Geometry: final body of the model. Coordinates: model frame, mm. Face numbers are marked on the shaded views. Give positions to 0.01 mm unless a question says otherwise; leave off trailing zeros. Write each loop counter-clockwise with the first axis right and the second up, starting at its lowest first coordinate (ties: lowest second). Pieces come first, ordered by that corner, then holes. Notation, with made-up numbers: (-34.75, -31) - (-2.75, -31) arc R22 ccw to (-2.75, -8) - close; hole circle Ø3 at (-26, 34). An arc over 180 degrees is marked (long way). Use CSV: the item, a comma, the result in double quotes. Start each with the question number.
(1) Section C-C on z = -36. Output: boundary loops of the cut face in (x, y), and give its area (3 significant figures).
(2) Draft query along Z for the marked faces 1 and 2. Return one class per face: released by +Z, released by -Z, zero draft, split by the parting line, or undercut.
(3) Section A-A on z = -1. Output: boundary loops of the cut face in (x, y), and give its area (3 significant figures).
(4) First-contact query: pin 1 Ø16 at (x, z) = (-97.5, -47) entering from +Y; pin 2 Ø3.5 at (x, z) = (-100, -71) entering from -Y; pin 3 Ø6.5 at (x, z) = (-92, -43.5) entering from +Y; pin 4 Ø5 at (x, z) = (-98.5, -71.5) entering from -Y. Flat tips, straight axial feed; report the tip coordinate or a pass-through.
(5) Line query: probe 1 along X at (y, z) = (-0.15, -71); probe 2 along X at (y, z) = (0.15, -45); probe 3 along Z at (x, y) = (-100, 0.1). Output: solid intervals per line, ascending. Write a range as [from, to].
(6) Section B-B on x = -1. Output: boundary loops of the cut face in (y, z), and give its area (3 significant figures).
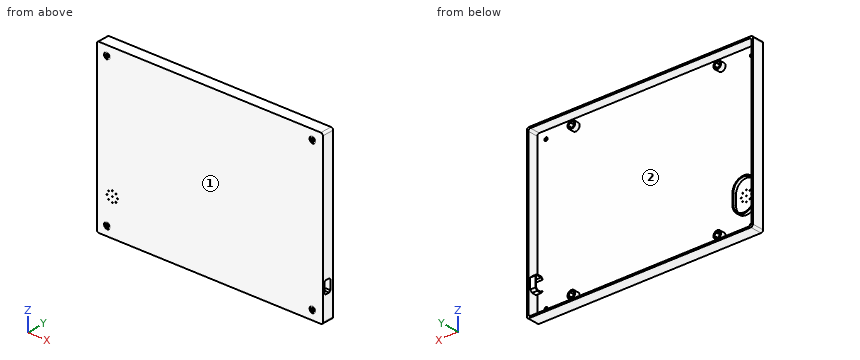
from build123d import *

# Parameters (mm, degrees)
EXTRUDE_1_DEPTH                 = 1
EXTRUDE_1_DEPTH_BACK            = 0.5
SKETCH_1_W                      = 220
SKETCH_1_H                      = 160
SKETCH_2_R                      = 3.75
EXTRUDE_2_DEPTH                 = 5
CUT_EXTRUDE_5_REACH             = 138.17
SKETCH_3_R                      = 1.6
CUT_EXTRUDE_5_DIRECTION_2_DEPTH = 137.169930601
CUT_EXTRUDE_START               = -0.5
SKETCH_4_R                      = 3
CUT_EXTRUDE_7_DEPTH             = 0.5
SKETCH_5_W                      = 220
SKETCH_5_H                      = 160
SKETCH_5_W_2                    = 217
SKETCH_5_H_2                    = 157
EXTRUDE_3_DEPTH                 = 10
FILLET_1_R                      = 2
FILLET_2_R                      = 2
FILLET_3_R                      = 2
CUT_EXTRUDE_8_REACH             = 236.352
CUT_EXTRUDE_8_DIRECTION_2_DEPTH = 235.352298901
EXTRUDE_4_DEPTH                 = 5
EXTRUDE_5_DEPTH                 = 3
CUT_EXTRUDE_9_REACH             = 138.382
SKETCH_10_R                     = 0.5


with BuildPart() as part:
    # 草图1 → 凸台-拉伸1 (new, two sides: drawn at the far end of the back side and taken through both)
    with BuildSketch(Plane(origin=(0, 0, 0), x_dir=(1, 0, 0), z_dir=(0, 1, 0)).offset(-EXTRUDE_1_DEPTH_BACK)):
        Rectangle(SKETCH_1_W, SKETCH_1_H)
    extrude(amount=EXTRUDE_1_DEPTH + EXTRUDE_1_DEPTH_BACK)

    # 草图2 → 凸台-拉伸2 (add)
    # profile 1 of 4: a face of its own
    with BuildSketch(Plane(origin=(0, 1, 0), x_dir=(1, 0, 0), z_dir=(0, 1, 0))):
        with Locations(Location((-71, 71, 0), (0, 0, 270))):
            Circle(SKETCH_2_R)
        Polygon((-69.614359354, 68.6), (-68.228718708, 71), (-69.614359354, 73.4), (-72.385640646, 73.4), (-73.771281292, 71), (-72.385640646, 68.6), align=None, mode=Mode.SUBTRACT)
    # profile 2 of 4: a face of its own
    with BuildSketch(Plane(origin=(0, 1, 0), x_dir=(1, 0, 0), z_dir=(0, 1, 0))):
        with Locations(Location((71, 71, 0), (0, 0, 90))):
            Circle(SKETCH_2_R)
        Polygon((72.385640646, 68.6), (69.614359354, 68.6), (68.228718708, 71), (69.614359354, 73.4), (72.385640646, 73.4), (73.771281292, 71), align=None, mode=Mode.SUBTRACT)
    # profile 3 of 4: a face of its own
    with BuildSketch(Plane(origin=(0, 1, 0), x_dir=(1, 0, 0), z_dir=(0, 1, 0))):
        with Locations(Location((71, -71, 0), (0, 0, 270))):
            Circle(SKETCH_2_R)
        Polygon((69.614359354, -68.6), (68.228718708, -71), (69.614359354, -73.4), (72.385640646, -73.4), (73.771281292, -71), (72.385640646, -68.6), align=None, mode=Mode.SUBTRACT)
    # profile 4 of 4: a face of its own
    with BuildSketch(Plane(origin=(0, 1, 0), x_dir=(1, 0, 0), z_dir=(0, 1, 0))):
        with Locations(Location((-71, -71, 0), (0, 0, 90))):
            Circle(SKETCH_2_R)
        Polygon((-72.385640646, -68.6), (-69.614359354, -68.6), (-68.228718708, -71), (-69.614359354, -73.4), (-72.385640646, -73.4), (-73.771281292, -71), align=None, mode=Mode.SUBTRACT)
    extrude(amount=EXTRUDE_2_DEPTH)

    # 草图3 → 切除-拉伸5 (cut, up to next)
    with BuildSketch(Plane.XZ.offset(0.5), mode=Mode.PRIVATE) as cut_extrude_5_sk1:
        with Locations(Location((-100, -71, 0), (0, 0, 90))):
            Circle(SKETCH_3_R)
    cut_extrude_5_tool1 = extrude(cut_extrude_5_sk1.sketch, amount=-CUT_EXTRUDE_5_REACH, mode=Mode.PRIVATE) & part.part
    # 草图3 → 切除-拉伸5 (cut, up to next)
    with BuildSketch(Plane.XZ.offset(0.5), mode=Mode.PRIVATE) as cut_extrude_5_sk2:
        with Locations(Location((100, -71, 0), (0, 0, 90))):
            Circle(SKETCH_3_R)
    cut_extrude_5_tool2 = extrude(cut_extrude_5_sk2.sketch, amount=-CUT_EXTRUDE_5_REACH, mode=Mode.PRIVATE) & part.part
    # 草图3 → 切除-拉伸5 (cut, up to next)
    with BuildSketch(Plane.XZ.offset(0.5), mode=Mode.PRIVATE) as cut_extrude_5_sk3:
        with Locations(Location((100, 71, 0), (0, 0, 90))):
            Circle(SKETCH_3_R)
    cut_extrude_5_tool3 = extrude(cut_extrude_5_sk3.sketch, amount=-CUT_EXTRUDE_5_REACH, mode=Mode.PRIVATE) & part.part
    # 草图3 → 切除-拉伸5 (cut, up to next)
    with BuildSketch(Plane.XZ.offset(0.5), mode=Mode.PRIVATE) as cut_extrude_5_sk4:
        with Locations(Location((-100, 71, 0), (0, 0, 90))):
            Circle(SKETCH_3_R)
    cut_extrude_5_tool4 = extrude(cut_extrude_5_sk4.sketch, amount=-CUT_EXTRUDE_5_REACH, mode=Mode.PRIVATE) & part.part
    add(cut_extrude_5_tool1.solids().sort_by_distance((-100, -0.5, -71))[0], mode=Mode.SUBTRACT)
    add(cut_extrude_5_tool2.solids().sort_by_distance((100, -0.5, -71))[0], mode=Mode.SUBTRACT)
    add(cut_extrude_5_tool3.solids().sort_by_distance((100, -0.5, 71))[0], mode=Mode.SUBTRACT)
    add(cut_extrude_5_tool4.solids().sort_by_distance((-100, -0.5, 71))[0], mode=Mode.SUBTRACT)

    # 草图3 → 切除-拉伸5 direction 2 (cut)
    with BuildSketch(Plane.XZ.offset(0.5)):
        with Locations(Location((-100, -71, 0), (0, 0, 90))):
            Circle(SKETCH_3_R)
        with Locations(Location((100, -71, 0), (0, 0, 90))):
            Circle(SKETCH_3_R)
        with Locations(Location((100, 71, 0), (0, 0, 90))):
            Circle(SKETCH_3_R)
        with Locations(Location((-100, 71, 0), (0, 0, 90))):
            Circle(SKETCH_3_R)
    extrude(amount=CUT_EXTRUDE_5_DIRECTION_2_DEPTH, mode=Mode.SUBTRACT)

    # 草图4 → 切除-拉伸7 (cut)
    with BuildSketch(Plane(origin=(0, 0, 0), x_dir=(1, 0, 0), z_dir=(0, 1, 0)).offset(CUT_EXTRUDE_START)):
        with Locations(Location((-100, 71, 0), (0, 0, 270))):
            Circle(SKETCH_4_R)
        with Locations(Location((100, 71, 0), (0, 0, 90))):
            Circle(SKETCH_4_R)
        with Locations(Location((100, -71, 0), (0, 0, 270))):
            Circle(SKETCH_4_R)
        with Locations(Location((-100, -71, 0), (0, 0, 90))):
            Circle(SKETCH_4_R)
    extrude(amount=CUT_EXTRUDE_7_DEPTH, mode=Mode.SUBTRACT)

    # 草图5 → 凸台-拉伸3 (add)
    with BuildSketch(Plane(origin=(0, 1, 0), x_dir=(1, 0, 0), z_dir=(0, 1, 0))):
        Rectangle(SKETCH_5_W, SKETCH_5_H)
        Rectangle(SKETCH_5_W_2, SKETCH_5_H_2, mode=Mode.SUBTRACT)
    extrude(amount=EXTRUDE_3_DEPTH)

    # 圆角1
    fillet_1_edges = [part.edges().sort_by_distance(p)[0] for p in [
        (-110, 5.25, -80),
    ]]
    fillet(fillet_1_edges, radius=FILLET_1_R)

    # 圆角2
    fillet_2_edges = [part.edges().sort_by_distance(p)[0] for p in [
        (-108.5, 6, -78.5),
    ]]
    fillet(fillet_2_edges, radius=FILLET_2_R)

    # 圆角3
    fillet_3_edges = [part.edges().sort_by_distance(p)[0] for p in [
        (108.5, 6, 78.5),
        (108.5, 6, -78.5),
        (-108.5, 6, 78.5),
        (110, 5.25, 80),
        (-110, 5.25, 80),
        (110, 5.25, -80),
    ]]
    fillet(fillet_3_edges, radius=FILLET_3_R)

    # 草图7 → 切除-拉伸8 (cut, up to next)
    with BuildSketch(Plane(origin=(110, 0, 0), x_dir=(0, 0, -1), z_dir=(1, 0, 0)), mode=Mode.PRIVATE) as cut_extrude_8_sk1:
        Polygon((45.435952693, 8), (54.607525568, 8), (56.02173913, 6.585786438), (56.02173913, 2.414213562), (54.607525568, 1), (45.435952693, 1), (44.02173913, 2.414213562), (44.02173913, 6.585786438), align=None)
    cut_extrude_8_tool1 = extrude(cut_extrude_8_sk1.sketch, amount=-CUT_EXTRUDE_8_REACH, mode=Mode.PRIVATE) & part.part
    add(cut_extrude_8_tool1.solids().sort_by_distance((110, 4.5, -50.021739))[0], mode=Mode.SUBTRACT)

    # 草图7 → 切除-拉伸8 direction 2 (cut)
    with BuildSketch(Plane(origin=(110, 0, 0), x_dir=(0, 0, -1), z_dir=(1, 0, 0))):
        Polygon((45.435952693, 8), (54.607525568, 8), (56.02173913, 6.585786438), (56.02173913, 2.414213562), (54.607525568, 1), (45.435952693, 1), (44.02173913, 2.414213562), (44.02173913, 6.585786438), align=None)
    extrude(amount=CUT_EXTRUDE_8_DIRECTION_2_DEPTH, mode=Mode.SUBTRACT)

    # 草图8 → 凸台-拉伸4 (add)
    with BuildSketch(Plane.ZY.offset(-108.5)):
        Polygon((-44.435952693, 1), (-43.02173913, 2.414213562), (-43.02173913, 7), (-45.02173913, 9), (-55.02173913, 9), (-57.02173913, 7), (-57.02173913, 2.414213562), (-55.607525568, 1), (-54.607525568, 1), (-56.02173913, 2.414213562), (-56.02173913, 6.585786438), (-54.607525568, 8), (-45.435952693, 8), (-44.02173913, 6.585786438), (-44.02173913, 2.414213562), (-45.435952693, 1), align=None)
    extrude(amount=EXTRUDE_4_DEPTH)

    # 草图9 → 凸台-拉伸5 (add)
    with BuildSketch(Plane(origin=(0, 1, 0), x_dir=(1, 0, 0), z_dir=(0, 1, 0))):
        with BuildLine():
            Line((-84, 50), (-84, 40))
            ThreePointArc((-84, 40), (-95, 29), (-106, 40))
            Line((-106, 40), (-106, 50))
            ThreePointArc((-106, 50), (-95, 61), (-84, 50))
        make_face()
        with BuildLine():
            Line((-85, 50), (-85, 40))
            ThreePointArc((-85, 40), (-95, 30), (-105, 40))
            Line((-105, 40), (-105, 50))
            ThreePointArc((-105, 50), (-95, 60), (-85, 50))
        make_face(mode=Mode.SUBTRACT)
    extrude(amount=EXTRUDE_5_DEPTH)

    # 草图10 → 切除-拉伸9 (cut, up to next)
    with BuildSketch(Plane(origin=(0, 1, 0), x_dir=(1, 0, 0), z_dir=(0, 1, 0)), mode=Mode.PRIVATE) as cut_extrude_9_sk1:
        with Locations(Location((-95, 45, 0), (0, 0, 270))):
            Circle(SKETCH_10_R)
    cut_extrude_9_tool1 = extrude(cut_extrude_9_sk1.sketch, amount=-CUT_EXTRUDE_9_REACH, mode=Mode.PRIVATE) & part.part
    # 草图10 → 切除-拉伸9 (cut, up to next)
    with BuildSketch(Plane(origin=(0, 1, 0), x_dir=(1, 0, 0), z_dir=(0, 1, 0)), mode=Mode.PRIVATE) as cut_extrude_9_sk2:
        with Locations(Location((-100, 45, 0), (0, 0, 270))):
            Circle(SKETCH_10_R)
    cut_extrude_9_tool2 = extrude(cut_extrude_9_sk2.sketch, amount=-CUT_EXTRUDE_9_REACH, mode=Mode.PRIVATE) & part.part
    # 草图10 → 切除-拉伸9 (cut, up to next)
    with BuildSketch(Plane(origin=(0, 1, 0), x_dir=(1, 0, 0), z_dir=(0, 1, 0)), mode=Mode.PRIVATE) as cut_extrude_9_sk3:
        with Locations(Location((-98.535533906, 48.535533906, 0), (0, 0, 270))):
            Circle(SKETCH_10_R)
    cut_extrude_9_tool3 = extrude(cut_extrude_9_sk3.sketch, amount=-CUT_EXTRUDE_9_REACH, mode=Mode.PRIVATE) & part.part
    # 草图10 → 切除-拉伸9 (cut, up to next)
    with BuildSketch(Plane(origin=(0, 1, 0), x_dir=(1, 0, 0), z_dir=(0, 1, 0)), mode=Mode.PRIVATE) as cut_extrude_9_sk4:
        with Locations(Location((-95, 50, 0), (0, 0, 270))):
            Circle(SKETCH_10_R)
    cut_extrude_9_tool4 = extrude(cut_extrude_9_sk4.sketch, amount=-CUT_EXTRUDE_9_REACH, mode=Mode.PRIVATE) & part.part
    # 草图10 → 切除-拉伸9 (cut, up to next)
    with BuildSketch(Plane(origin=(0, 1, 0), x_dir=(1, 0, 0), z_dir=(0, 1, 0)), mode=Mode.PRIVATE) as cut_extrude_9_sk5:
        with Locations(Location((-91.464466094, 48.535533906, 0), (0, 0, 270))):
            Circle(SKETCH_10_R)
    cut_extrude_9_tool5 = extrude(cut_extrude_9_sk5.sketch, amount=-CUT_EXTRUDE_9_REACH, mode=Mode.PRIVATE) & part.part
    # 草图10 → 切除-拉伸9 (cut, up to next)
    with BuildSketch(Plane(origin=(0, 1, 0), x_dir=(1, 0, 0), z_dir=(0, 1, 0)), mode=Mode.PRIVATE) as cut_extrude_9_sk6:
        with Locations(Location((-90, 45, 0), (0, 0, 270))):
            Circle(SKETCH_10_R)
    cut_extrude_9_tool6 = extrude(cut_extrude_9_sk6.sketch, amount=-CUT_EXTRUDE_9_REACH, mode=Mode.PRIVATE) & part.part
    # 草图10 → 切除-拉伸9 (cut, up to next)
    with BuildSketch(Plane(origin=(0, 1, 0), x_dir=(1, 0, 0), z_dir=(0, 1, 0)), mode=Mode.PRIVATE) as cut_extrude_9_sk7:
        with Locations(Location((-91.464466094, 41.464466094, 0), (0, 0, 270))):
            Circle(SKETCH_10_R)
    cut_extrude_9_tool7 = extrude(cut_extrude_9_sk7.sketch, amount=-CUT_EXTRUDE_9_REACH, mode=Mode.PRIVATE) & part.part
    # 草图10 → 切除-拉伸9 (cut, up to next)
    with BuildSketch(Plane(origin=(0, 1, 0), x_dir=(1, 0, 0), z_dir=(0, 1, 0)), mode=Mode.PRIVATE) as cut_extrude_9_sk8:
        with Locations(Location((-95, 40, 0), (0, 0, 270))):
            Circle(SKETCH_10_R)
    cut_extrude_9_tool8 = extrude(cut_extrude_9_sk8.sketch, amount=-CUT_EXTRUDE_9_REACH, mode=Mode.PRIVATE) & part.part
    # 草图10 → 切除-拉伸9 (cut, up to next)
    with BuildSketch(Plane(origin=(0, 1, 0), x_dir=(1, 0, 0), z_dir=(0, 1, 0)), mode=Mode.PRIVATE) as cut_extrude_9_sk9:
        with Locations(Location((-98.535533906, 41.464466094, 0), (0, 0, 270))):
            Circle(SKETCH_10_R)
    cut_extrude_9_tool9 = extrude(cut_extrude_9_sk9.sketch, amount=-CUT_EXTRUDE_9_REACH, mode=Mode.PRIVATE) & part.part
    add(cut_extrude_9_tool1.solids().sort_by_distance((-95, 1, -45))[0], mode=Mode.SUBTRACT)
    add(cut_extrude_9_tool2.solids().sort_by_distance((-100, 1, -45))[0], mode=Mode.SUBTRACT)
    add(cut_extrude_9_tool3.solids().sort_by_distance((-98.535534, 1, -48.535534))[0], mode=Mode.SUBTRACT)
    add(cut_extrude_9_tool4.solids().sort_by_distance((-95, 1, -50))[0], mode=Mode.SUBTRACT)
    add(cut_extrude_9_tool5.solids().sort_by_distance((-91.464466, 1, -48.535534))[0], mode=Mode.SUBTRACT)
    add(cut_extrude_9_tool6.solids().sort_by_distance((-90, 1, -45))[0], mode=Mode.SUBTRACT)
    add(cut_extrude_9_tool7.solids().sort_by_distance((-91.464466, 1, -41.464466))[0], mode=Mode.SUBTRACT)
    add(cut_extrude_9_tool8.solids().sort_by_distance((-95, 1, -40))[0], mode=Mode.SUBTRACT)
    add(cut_extrude_9_tool9.solids().sort_by_distance((-98.535534, 1, -41.464466))[0], mode=Mode.SUBTRACT)


solid = part.part
Check values:
1,outline,"(-110, -0.5) - (110, -0.5) - (110, 11) - (108.5, 11) - (108.5, 1) - (-84.75, 1) - (-84.75, 4) - (-85.83, 4) - (-85.83, 1) - (-104.17, 1) - (-104.17, 4) - (-105.25, 4) - (-105.25, 1) - (-108.5, 1) - (-108.5, 11) - (-110, 11) - close"
1,area,"366 mm²"
2,face 1,"zero draft"
2,face 2,"undercut"
3,outline,"(-110, -0.5) - (110, -0.5) - (110, 11) - (108.5, 11) - (108.5, 1) - (-108.5, 1) - (-108.5, 11) - (-110, 11) - close"
3,area,"360 mm²"
4,pin 1,"stops at y = 4"
4,pin 2,"stops at y = 0"
4,pin 3,"stops at y = 1"
4,pin 4,"stops at y = -0.5"
5,probe 1,"x = [-110, -103], [-97, 97], [103, 110]"
5,probe 2,"x = [-110, -100.5], [-99.5, -95.5], [-94.5, -90.5], [-89.5, 110]"
5,probe 3,"z = [-80, -72.6], [-69.4, -45.5], [-44.5, 69.4], [72.6, 80]"
6,outline,"(-0.5, -80) - (11, -80) - (11, -78.5) - (1, -78.5) - (1, 78.5) - (11, 78.5) - (11, 80) - (-0.5, 80) - close"
6,area,"270 mm²"
